from build123d import *

# Parameters (mm, degrees)
F0_W     = 15
F0_H     = 5
F0_R     = 1.25
F1_DEPTH = 15
F3_D     = 2.5


with BuildPart() as f1:
    # F0 (on Top) → F1 (new body)
    with BuildSketch(Plane.XY):
        Rectangle(F0_W, F0_H)
        with Locations((-5, 0)):
            Circle(F0_R, mode=Mode.SUBTRACT)
        with Locations((5, 0)):
            Circle(F0_R, mode=Mode.SUBTRACT)
    extrude(amount=F1_DEPTH)

    # F3 (through all)
    with Locations(Plane.XZ.offset(2.5)):
        with Locations((0.5, 11.5), (-5, 7.5), (0.5, 3.5)):
            Hole(F3_D / 2)


solid = f1.part
Can you work these out from the model? Positions are in its coordinate system, mm. Round coordinates to 2 decimals unless told otherwise and drop trailing zeros. Order: outer loops, then holes, each group sorted by start corner. A loop starts at its lowest first (then second) coordinate and runs counter-clockwise, first axis right, second up. Notation, with made-up numbers: M 27.25,52 L 67.25,52 A17 cw 67.25,63 Z; hole C 17.5,22.5 d7. An arc over 180 degrees is marked long. Use a Markdown table: item, result.
1) If I drill on line 1 along X through (y, z) = (0.1, 1); line 2 along Z through (x, y) = (0.5, -0.3); line 3 along Z through (x, y) = (-5, -1.4), over which ranges is the centre line in solid material (lowest first)?
Geometry says:
| item | result |
|---|---|
| line 1 | x = -7.5 to -6.25, -3.75 to 3.75, 6.25 to 7.5 |
| line 2 | z = 0 to 2.25, 4.75 to 10.25, 12.75 to 15 |
| line 3 | z = 0 to 6.25, 8.75 to 15 |
2) Imagine slicing it at D-D (x = 0.5). List the corners of the cut face in (y, z) for me.
Geometry says:
| item | result |
|---|---|
| outline | M -2.5,0 L 2.5,0 L 2.5,2.25 L -2.5,2.25 Z; M -2.5,4.75 L 2.5,4.75 L 2.5,10.25 L -2.5,10.25 Z; M -2.5,12.75 L 2.5,12.75 L 2.5,15 L -2.5,15 Z |
3) Imagine slicing it at A-A (x = 5). List the corners of the cut face in (y, z) for me.
Geometry says:
| item | result |
|---|---|
| outline | M -2.5,0 L -1.25,0 L -1.25,15 L -2.5,15 Z; M 1.25,0 L 2.5,0 L 2.5,15 L 1.25,15 Z |
4) I'm going to push a flat-ended pin straight in: P1, Ø2, axis at x = -5, z = 7.5, coming from the -Y side. Where does the tip first touch, or does it pass through?
Geometry says:
| item | result |
|---|---|
| P1 | passes through |
5) Imagine slicing it at C-C (y = -0.9). List the corners of the cut face in (x, z) for me.
Geometry says:
| item | result |
|---|---|
| outline | M -7.5,0 L -5.87,0 L -5.87,6.6 A1.25 cw -5.87,8.4 L -5.87,15 L -7.5,15 Z; M -4.13,0 L 4.13,0 L 4.13,15 L -4.13,15 L -4.13,8.4 A1.25 cw -4.13,6.6 Z; M 5.87,0 L 7.5,0 L 7.5,15 L 5.87,15 Z; hole C 0.5,3.5 d2.5; hole C 0.5,11.5 d2.5 |
6) Imagine slicing it at B-B (z = 11.5). List the corners of the cut face in (x, y) for me.
Geometry says:
| item | result |
|---|---|
| outline | M -7.5,-2.5 L -0.75,-2.5 L -0.75,2.5 L -7.5,2.5 Z; M 1.75,-2.5 L 7.5,-2.5 L 7.5,2.5 L 1.75,2.5 Z; hole C -5,0 d2.5; hole C 5,0 d2.5 |
7) If we mould it in two halves opening along Z, with no side actions, what happens to faces 1 (the face through (7.5, 0, 7)), 2 (the face through (0.77, 0.04, 2.28)), 3 (the face through (0, 0, 0))? For each: +Z half, -Z half, draft (parallel to the pull), parting line (faces both ways), or undercut.
Geometry says:
| item | result |
|---|---|
| face 1 | draft |
| face 2 | undercut |
| face 3 | -Z half |
